Source: CAD feature listing. Evaluate the final solid. Frame: model axes, mm. Face numbers are marked on the shaded views. Round coordinates to 2 decimals unless told otherwise and drop trailing zeros. Loops run counter-clockwise (first coordinate to the right, second up) from the corner with the lowest first, then second, coordinate; pieces in that order, holes last. Notation, with made-up numbers: (-5.75, -28) -> (10.25, -28) arc R26 ccw to (10.25, 4) -> close; hole circle Ø11 at (35.25, -26). An arc over 180 degrees is marked (long way). Put each result on its own line as item: value. Start each with the question number.
1. Cut plane D-D (x = 175). Return the cut outline in (y, z), then the cut area to 3 significant figures.
2. Draft query along X for the marked faces 1 and 2. Return one class per face: pulls with the +X half, pulls with the -X half, needs draft (parallel to the pull), parting line crosses it, or undercut.
3. Cut plane B-B (z = -58). Return the cut outline in (x, y).
4. Material intervals for L1, parallel to X at y = 4.25, z = -49; L2, parallel to Z at x = 180, y = 0.5; L3, parallel to X at y = 8.75, z = -58, sorted ascending.
5. Contact query for flat-ended pins moving along their axis: pin 1 (1.6 mm diameter, centred on y = 10, z = -43, fed in from -X); pin 2 (6 mm diameter, centred on x = 84.5, y = 6.5, fed in from -Z); pin 3 (0.6 mm diameter, centred on x = 212, y = 11, fed in from +Z). Output: stop coordinate, or through.
6. Cut plane A-A (x = 225). Return the cut outline in (y, z) (3 decimals), then the cut area to 3 significant figures.
```python
from build123d import *

# Parameters (mm, degrees)
SKETCH1_W              = 260
SKETCH1_H              = 116
BOSS_EXTRUDE1_DEPTH    = 11.62
FILLET1_R              = 5
FILLET2_R              = 3
SKETCH2_W              = 254
SKETCH2_H              = 110
CUT_EXTRUDE1_DEPTH     = 8.62
FILLET3_R              = 3
SKETCH6_R              = 9.3599
CUT_EXTRUDE4_DEPTH     = 8.636
SKETCH7_W              = 51
SKETCH7_H              = 15.649055797
BOSS_EXTRUDE3_DEPTH    = 3
FILLET6_R              = 8
FILLET7_R              = 8
SKETCH8_W              = 51
SKETCH8_H              = 3
BOSS_EXTRUDE4_DEPTH    = 1.5
CUT_EXTRUDE5_DEPTH     = 55
LPATTERN2_COUNT        = 2
LPATTERN2_PITCH        = 161
FILLET6_OF_LPATTERN2_R = 8
FILLET7_OF_LPATTERN2_R = 8
SKETCH10_W             = 51
SKETCH10_H             = 15.62
BOSS_EXTRUDE5_DEPTH    = 3
FILLET8_R              = 8
SKETCH11_W             = 51
SKETCH11_H             = 3
BOSS_EXTRUDE6_DEPTH    = 1.5
CUT_EXTRUDE6_DEPTH     = 55
LPATTERN3_COUNT        = 2
LPATTERN3_PITCH        = 161
FILLET8_OF_LPATTERN3_R = 8
CHAMFER1_SIZE          = 15
CHAMFER1_SIZE2         = 2.644904711
SKETCH13_W             = 18.833961405
SKETCH13_H             = 27.155748893
SKETCH13_W_2           = 23.540134481
SKETCH13_H_2           = 26.001362064
SKETCH13_W_3           = 13.410899097
SKETCH13_H_3           = 18.756893662
SKETCH13_W_4           = 15.344585033
SKETCH13_H_4           = 16.316593901
BOSS_EXTRUDE7_DEPTH    = 3


with BuildPart() as part:
    # Sketch1 → Boss-Extrude1 (new body)
    with BuildSketch(Plane(origin=(0, 0, 0), x_dir=(1, 0, 0), z_dir=(0, 1, 0))):
        with Locations((130, 58)):
            Rectangle(SKETCH1_W, SKETCH1_H)
    extrude(amount=BOSS_EXTRUDE1_DEPTH)

    # Fillet1
    fillet1_edges = [part.edges().sort_by_distance(p)[0] for p in [
        (0, 5.81, -116),
        (260, 5.81, -116),
        (260, 5.81, 0),
        (0, 5.81, 0),
    ]]
    fillet(fillet1_edges, radius=FILLET1_R)

    # Fillet2
    fillet2_edges = [part.edges().sort_by_distance(p)[0] for p in [
        (130, 11.62, 0),
        (0, 11.62, -58),
        (260, 11.62, -58),
        (130, 11.62, -116),
        (1.464466094, 11.62, -114.535533906),
        (258.535533906, 11.62, -114.535533906),
        (258.535533906, 11.62, -1.464466094),
        (1.464466094, 11.62, -1.464466094),
    ]]
    fillet(fillet2_edges, radius=FILLET2_R)

    # Sketch2 → Cut-Extrude1 (cut)
    with BuildSketch(Plane.XZ):
        with Locations((130, -58)):
            Rectangle(SKETCH2_W, SKETCH2_H)
    extrude(amount=-CUT_EXTRUDE1_DEPTH, mode=Mode.SUBTRACT)

    # Fillet3
    fillet3_edges = [part.edges().sort_by_distance(p)[0] for p in [
        (3, 4.31, -113),
        (3, 4.31, -3),
        (257, 4.31, -3),
        (257, 4.31, -113),
    ]]
    fillet(fillet3_edges, radius=FILLET3_R)

    # Sketch6 → Cut-Extrude4 (cut)
    with BuildSketch(Plane(origin=(0, 11.62, 0), x_dir=(1, 0, 0), z_dir=(0, 1, 0))):
        with Locations(Location((225, 58, 0), (0, 0, 270))):
            Circle(SKETCH6_R)
    extrude(amount=-CUT_EXTRUDE4_DEPTH, mode=Mode.SUBTRACT)

    # Sketch7 → Boss-Extrude3 (add)
    with BuildSketch(Plane.XY):
        with Locations((49.5, 0.824527899)):
            Rectangle(SKETCH7_W, SKETCH7_H)
    boss_extrude3 = extrude(amount=BOSS_EXTRUDE3_DEPTH)

    # Fillet6
    # the kernel refuses this fillet: 8 mm, written as the material it takes off along each edge
    with BuildSketch(Plane(origin=(8.387505004, 8.649055797, 3), x_dir=(0, 0, -1), z_dir=(1, 0, 0))) as fillet6_piece_1:
        with BuildLine():
            CenterArc((8, -6.244997998), FILLET6_R, 128.682187453, 51.317812547)
            Line((0, -6.244997998), (-0.16, -6.244997998))
            Line((-0.16, -6.244997998), (-0.16, 0))
            Line((-0.16, 0), (0, 0.16))
            ThreePointArc((0, 0.16), (1.5, 0.16), (2.9, 0.12489996))
            Line((2.9, 0.12489996), (3, 0))
        make_face()
    extrude(amount=82.224989992, mode=Mode.SUBTRACT)

    # Fillet7
    # the kernel refuses this fillet: 8 mm, written as the material it takes off along each edge
    with BuildSketch(Plane(origin=(90.612494996, -7, 3), x_dir=(0, 0, -1), z_dir=(-1, 0, 0))) as fillet7_piece_1:
        with BuildLine():
            CenterArc((8, -6.244997998), FILLET7_R, 128.682187453, 51.317812547)
            Line((0, -6.244997998), (-0.16, -6.244997998))
            Line((-0.16, -6.244997998), (-0.16, 0))
            Line((-0.16, 0), (0, 0.16))
            ThreePointArc((0, 0.16), (1.5, 0.16), (2.9, 0.12489996))
            Line((2.9, 0.12489996), (3, 0))
        make_face()
    extrude(amount=82.224989992, mode=Mode.SUBTRACT)

    # Sketch8 → Boss-Extrude4 (add)
    with BuildSketch(Plane(origin=(0, 0, 0), x_dir=(-1, 0, 0), z_dir=(0, 0, -1))):
        with Locations((-49.5, -5.5)):
            Rectangle(SKETCH8_W, SKETCH8_H)
    boss_extrude4 = extrude(amount=BOSS_EXTRUDE4_DEPTH)

    # Sketch9 → Cut-Extrude5 (cut)
    with BuildSketch(Plane.ZY.offset(-24)):
        Polygon((0, -4), (-1.5, -5.5), (0, -7), (-1.5, -7), (-2.053402402, -7), (-2.053402402, -4), (-1.5, -4), align=None)
    cut_extrude5 = extrude(amount=-CUT_EXTRUDE5_DEPTH, mode=Mode.SUBTRACT)

    # LPattern2: Boss-Extrude3, Boss-Extrude4, Cut-Extrude5 ×2
    with Locations(*[(i * LPATTERN2_PITCH, 0, 0) for i in range(1, LPATTERN2_COUNT)]):
        add(boss_extrude3)
        add(boss_extrude4)
        add(cut_extrude5, mode=Mode.SUBTRACT)

    # Fillet6 of LPattern2
    # the kernel refuses this fillet: 8 mm, written as the material it takes off along each edge
    with BuildSketch(Plane(origin=(169.387505004, 8.649055797, 3), x_dir=(0, 0, -1), z_dir=(1, 0, 0))) as fillet6_of_lpattern2_piece_1:
        with BuildLine():
            CenterArc((8, -6.244997998), FILLET6_OF_LPATTERN2_R, 128.682187453, 51.317812547)
            Line((0, -6.244997998), (-0.16, -6.244997998))
            Line((-0.16, -6.244997998), (-0.16, 0))
            Line((-0.16, 0), (0, 0.16))
            ThreePointArc((0, 0.16), (1.5, 0.16), (2.9, 0.12489996))
            Line((2.9, 0.12489996), (3, 0))
        make_face()
    extrude(amount=82.224989992, mode=Mode.SUBTRACT)

    # Fillet7 of LPattern2
    # the kernel refuses this fillet: 8 mm, written as the material it takes off along each edge
    with BuildSketch(Plane(origin=(251.612494996, -7, 3), x_dir=(0, 1, 0), z_dir=(-1, 0, 0))) as fillet7_of_lpattern2_piece_1:
        with BuildLine():
            CenterArc((6.244997998, 8), FILLET7_OF_LPATTERN2_R, 218.682187453, 51.317812547)
            Line((0, 3), (-0.12489996, 2.9))
            ThreePointArc((-0.12489996, 2.9), (-0.16, 1.5), (-0.16, 0))
            Line((-0.16, 0), (0, -0.16))
            Line((0, -0.16), (6.244997998, -0.16))
            Line((6.244997998, -0.16), (6.244997998, 0))
        make_face()
    extrude(amount=82.224989992, mode=Mode.SUBTRACT)

    # Sketch10 → Boss-Extrude5 (add)
    with BuildSketch(Plane(origin=(0, 0, -116), x_dir=(-1, 0, 0), z_dir=(0, 0, -1))):
        with Locations((-49.5, 0.81)):
            Rectangle(SKETCH10_W, SKETCH10_H)
    boss_extrude5 = extrude(amount=BOSS_EXTRUDE5_DEPTH)

    # Fillet8
    # the kernel refuses this fillet: 8 mm, written as the material it takes off along each edge
    with BuildSketch(Plane(origin=(8.387505004, -7, -119), x_dir=(0, 0, 1), z_dir=(1, 0, 0)), Plane(origin=(90.612494996, 8.62, -119), x_dir=(0, 0, 1), z_dir=(-1, 0, 0))) as fillet8_piece_1:
        with BuildLine():
            CenterArc((8, -6.244997998), FILLET8_R, 128.682187453, 51.317812547)
            Line((0, -6.244997998), (-0.16, -6.244997998))
            Line((-0.16, -6.244997998), (-0.16, 0))
            Line((-0.16, 0), (0, 0.16))
            ThreePointArc((0, 0.16), (1.5, 0.16), (2.9, 0.12489996))
            Line((2.9, 0.12489996), (3, 0))
        make_face()
    extrude(amount=82.224989992, mode=Mode.SUBTRACT)

    # Sketch11 → Boss-Extrude6 (add)
    with BuildSketch(Plane.XY.offset(-116)):
        with Locations((49.5, -5.5)):
            Rectangle(SKETCH11_W, SKETCH11_H)
    boss_extrude6 = extrude(amount=BOSS_EXTRUDE6_DEPTH)

    # Sketch12 → Cut-Extrude6 (cut)
    with BuildSketch(Plane.ZY.offset(-24)):
        Polygon((-116, -4), (-114.5, -5.5), (-116, -7), (-111.986018157, -7), (-111.986018157, -3.7983216), align=None)
    cut_extrude6 = extrude(amount=-CUT_EXTRUDE6_DEPTH, mode=Mode.SUBTRACT)

    # LPattern3: Boss-Extrude5, Boss-Extrude6, Cut-Extrude6 ×2
    with Locations(*[(i * LPATTERN3_PITCH, 0, 0) for i in range(1, LPATTERN3_COUNT)]):
        add(boss_extrude5)
        add(boss_extrude6)
        add(cut_extrude6, mode=Mode.SUBTRACT)

    # Fillet8 of LPattern3
    # the kernel refuses this fillet: 8 mm, written as the material it takes off along each edge
    with BuildSketch(Plane(origin=(169.387505004, -7, -119), x_dir=(0, 0, 1), z_dir=(1, 0, 0)), Plane(origin=(251.612494996, 8.62, -119), x_dir=(0, 0, 1), z_dir=(-1, 0, 0))) as fillet8_of_lpattern3_piece_1:
        with BuildLine():
            CenterArc((8, -6.244997998), FILLET8_OF_LPATTERN3_R, 128.682187453, 51.317812547)
            Line((0, -6.244997998), (-0.16, -6.244997998))
            Line((-0.16, -6.244997998), (-0.16, 0))
            Line((-0.16, 0), (0, 0.16))
            ThreePointArc((0, 0.16), (1.5, 0.16), (2.9, 0.12489996))
            Line((2.9, 0.12489996), (3, 0))
        make_face()
    extrude(amount=82.224989992, mode=Mode.SUBTRACT)

    # Chamfer1
    chamfer1_edges = [part.edges().sort_by_distance(p)[0] for p in [
        (225, 11.62, -67.3599),
    ]]
    chamfer1_side = [part.faces().sort_by_distance(p)[0] for p in [
        (129.054758669, 11.62, -58),
    ]]
    chamfer(chamfer1_edges, length=CHAMFER1_SIZE, length2=CHAMFER1_SIZE2, reference=chamfer1_side[0])

    # Sketch13 → Boss-Extrude7 (add)
    with BuildSketch(Plane(origin=(0, 11.62, 0), x_dir=(1, 0, 0), z_dir=(0, 1, 0))):
        with Locations((243.776980702, 80.937874447)):
            Rectangle(SKETCH13_W, SKETCH13_H)
        with Locations((203.86993276, 80.360681032)):
            Rectangle(SKETCH13_W_2, SKETCH13_H_2)
        with Locations((241.065449548, 39.261553169)):
            Rectangle(SKETCH13_W_3, SKETCH13_H_3)
        with Locations((207.967707484, 40.481703049)):
            Rectangle(SKETCH13_W_4, SKETCH13_H_4)
    extrude(amount=-BOSS_EXTRUDE7_DEPTH)


solid = part.part
```
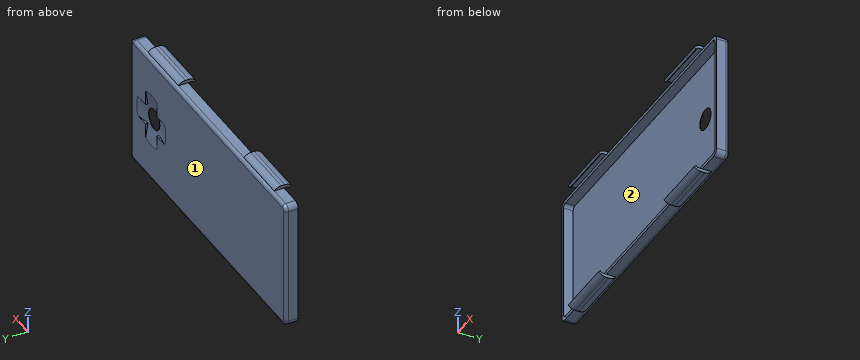
Solution:
1. outline: (0, -116) -> (8.62, -116) arc R3 ccw to (11.62, -113) -> (11.62, -3) arc R3 ccw to (8.62, 0) -> (0, 0) -> (0, -3) -> (8.62, -3) -> (8.62, -113) -> (0, -113) -> close
1. area: 396 mm^2
2. face 1: needs draft
2. face 2: undercut
3. outline: (0, 0) -> (3, 0) -> (3, 8.62) -> (215.64, 8.62) -> (215.64, 8.98) -> (200.64, 11.62) -> (3, 11.62) arc R3 ccw to (0, 8.62) -> close; (234.36, 8.62) -> (257, 8.62) -> (257, 0) -> (260, 0) -> (260, 8.62) arc R3 ccw to (257, 11.62) -> (249.36, 11.62) -> (234.36, 8.98) -> close
4. L1: x = 0 to 3, 257 to 260
4. L2: z = -116 to -113, -3 to 0
4. L3: x = 0 to 215.64, 234.36 to 260
5. pin 1: stops at x = 0.06
5. pin 2: stops at z = -116
5. pin 3: stops at z = -0.84
6. outline: (-7, -116) arc R8 ccw to (-0.755, -119) -> (2.375, -119) arc R8 ccw to (8.62, -116) arc R3 ccw to (11.62, -113) -> (11.62, -82.36) -> (8.975, -67.36) -> (8.62, -67.36) -> (8.62, -113) -> (0, -113) -> (0, -116) -> (-4, -116) -> (-5.5, -114.5) -> close; (-7, 0) -> (-5.5, -1.5) -> (-4, 0) -> (0, 0) -> (0, -3) -> (8.62, -3) -> (8.62, -48.64) -> (8.975, -48.64) -> (11.62, -33.64) -> (11.62, -3) arc R3 ccw to (8.62, 0) -> (8.649, 0) arc R8 ccw to (2.404, 3) -> (-0.755, 3) arc R8 ccw to start
6. area: 376 mm^2
